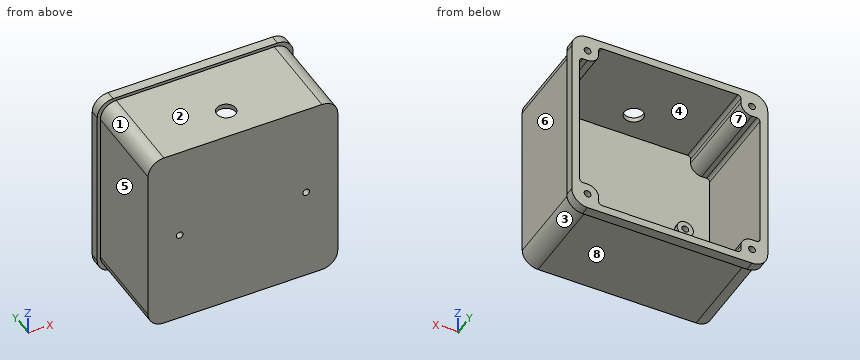
```python
from build123d import *

# Parameters (mm, degrees)
SKETCH1_W           = 120
SKETCH1_H           = 120
BOSS_EXTRUDE1_DEPTH = 63
SHELL1_T            = -3
SKETCH2_R           = 2.15
BOSS_EXTRUDE2_DEPTH = 60
SKETCH3_W           = 124
SKETCH3_H           = 124
SKETCH3_W_2         = 120
SKETCH3_H_2         = 120
BOSS_EXTRUDE3_DEPTH = 6
FILLET1_R           = 10
SKETCH4_R           = 2.15
CUT_EXTRUDE1_DEPTH  = 3
BOSS_EXTRUDE4_START = 3
SKETCH5_R           = 5.15
SKETCH5_R_2         = 2.15
BOSS_EXTRUDE4_DEPTH = 3
SKETCH6_R           = 6
CUT_EXTRUDE2_DEPTH  = 10


with BuildPart() as part:
    # Sketch1 → Boss-Extrude1 (new body)
    with BuildSketch(Plane(origin=(0, 0, 0), x_dir=(1, 0, 0), z_dir=(0, 1, 0))):
        Rectangle(SKETCH1_W, SKETCH1_H)
    extrude(amount=BOSS_EXTRUDE1_DEPTH)

    # Shell1
    shell1_openings = [part.faces().sort_by_distance(p)[0] for p in [
        (0, 63, 0),
    ]]
    offset(amount=SHELL1_T, openings=shell1_openings, kind=Kind.INTERSECTION)

    # Sketch2 → Boss-Extrude2 (add)
    # profile 1 of 4: a face of its own
    with BuildSketch(Plane(origin=(0, 3, 0), x_dir=(1, 0, 0), z_dir=(0, 1, 0))):
        with BuildLine():
            Line((52, 44.98), (55, 44.98))
            ThreePointArc((55, 44.98), (56.414213562, 44.394213562), (57, 42.98))
            Line((57, 42.98), (57, 57))
            Line((57, 57), (42.98, 57))
            ThreePointArc((42.98, 57), (44.394213562, 56.414213562), (44.98, 55))
            Line((44.98, 55), (44.98, 52))
            ThreePointArc((44.98, 52), (47.036110396, 47.036110396), (52, 44.98))
        make_face()
        with Locations(Location((52, 52, 0), (0, 0, 90))):
            Circle(SKETCH2_R, mode=Mode.SUBTRACT)
    # profile 2 of 4: a face of its own
    with BuildSketch(Plane(origin=(0, 3, 0), x_dir=(1, 0, 0), z_dir=(0, 1, 0))):
        with BuildLine():
            Line((-44.98, 52), (-44.98, 55))
            ThreePointArc((-44.98, 55), (-44.394213562, 56.414213562), (-42.98, 57))
            Line((-42.98, 57), (-57, 57))
            Line((-57, 57), (-57, 42.98))
            ThreePointArc((-57, 42.98), (-56.414213562, 44.394213562), (-55, 44.98))
            Line((-55, 44.98), (-52, 44.98))
            ThreePointArc((-52, 44.98), (-47.036110396, 47.036110396), (-44.98, 52))
        make_face()
        with Locations(Location((-52, 52, 0), (0, 0, 270))):
            Circle(SKETCH2_R, mode=Mode.SUBTRACT)
    # profile 3 of 4: a face of its own
    with BuildSketch(Plane(origin=(0, 3, 0), x_dir=(1, 0, 0), z_dir=(0, 1, 0))):
        with BuildLine():
            Line((57, -42.98), (57, -57))
            Line((57, -57), (42.98, -57))
            ThreePointArc((42.98, -57), (44.394213562, -56.414213562), (44.98, -55))
            Line((44.98, -55), (44.98, -52))
            ThreePointArc((44.98, -52), (47.036110396, -47.036110396), (52, -44.98))
            Line((52, -44.98), (55, -44.98))
            ThreePointArc((55, -44.98), (56.414213562, -44.394213562), (57, -42.98))
        make_face()
        with Locations(Location((52, -52, 0), (0, 0, 270))):
            Circle(SKETCH2_R, mode=Mode.SUBTRACT)
    # profile 4 of 4: a face of its own
    with BuildSketch(Plane(origin=(0, 3, 0), x_dir=(1, 0, 0), z_dir=(0, 1, 0))):
        with BuildLine():
            Line((-52, -44.98), (-55, -44.98))
            ThreePointArc((-55, -44.98), (-56.414213562, -44.394213562), (-57, -42.98))
            Line((-57, -42.98), (-57, -57))
            Line((-57, -57), (-42.98, -57))
            ThreePointArc((-42.98, -57), (-44.394213562, -56.414213562), (-44.98, -55))
            Line((-44.98, -55), (-44.98, -52))
            ThreePointArc((-44.98, -52), (-47.036110396, -47.036110396), (-52, -44.98))
        make_face()
        with Locations(Location((-52, -52, 0), (0, 0, 90))):
            Circle(SKETCH2_R, mode=Mode.SUBTRACT)
    extrude(amount=BOSS_EXTRUDE2_DEPTH)

    # Sketch3 → Boss-Extrude3 (add)
    with BuildSketch(Plane(origin=(0, 63, 0), x_dir=(1, 0, 0), z_dir=(0, 1, 0))):
        Rectangle(SKETCH3_W, SKETCH3_H)
        Rectangle(SKETCH3_W_2, SKETCH3_H_2, mode=Mode.SUBTRACT)
    extrude(amount=-BOSS_EXTRUDE3_DEPTH)

    # Fillet1
    fillet1_edges = [part.edges().sort_by_distance(p)[0] for p in [
        (60, 28.5, 60),
        (-60, 28.5, 60),
        (-60, 28.5, -60),
        (60, 28.5, -60),
        (62, 60, -62),
        (62, 60, 62),
        (-62, 60, 62),
        (-62, 60, -62),
    ]]
    fillet(fillet1_edges, radius=FILLET1_R)

    # Sketch4 → Cut-Extrude1 (cut)
    with BuildSketch(Plane(origin=(0, 3, 0), x_dir=(1, 0, 0), z_dir=(0, 1, 0))):
        with Locations(Location((-40, 0, 0), (0, 0, 270))):
            Circle(SKETCH4_R)
        with Locations(Location((40, 0, 0), (0, 0, 90))):
            Circle(SKETCH4_R)
    extrude(amount=-CUT_EXTRUDE1_DEPTH, mode=Mode.SUBTRACT)

    # Sketch5 → Boss-Extrude4 (add)
    # profile 1 of 2: a face of its own
    with BuildSketch(Plane(origin=(0, 3, 0), x_dir=(1, 0, 0), z_dir=(0, 1, 0)).offset(BOSS_EXTRUDE4_START)):
        with Locations(Location((-40, 0, 0), (0, 0, 270))):
            Circle(SKETCH5_R)
        with Locations(Location((-40, 0, 0), (0, 0, 270))):
            Circle(SKETCH5_R_2, mode=Mode.SUBTRACT)
    # profile 2 of 2: a face of its own
    with BuildSketch(Plane(origin=(0, 3, 0), x_dir=(1, 0, 0), z_dir=(0, 1, 0)).offset(BOSS_EXTRUDE4_START)):
        with Locations(Location((40, 0, 0), (0, 0, 90))):
            Circle(SKETCH5_R)
        with Locations(Location((40, 0, 0), (0, 0, 90))):
            Circle(SKETCH5_R_2, mode=Mode.SUBTRACT)
    extrude(amount=-BOSS_EXTRUDE4_DEPTH)

    # Sketch6 → Cut-Extrude2 (cut)
    with BuildSketch(Plane.XY.offset(60)):
        with Locations((0, 20)):
            Circle(SKETCH6_R)
    extrude(amount=-CUT_EXTRUDE2_DEPTH, mode=Mode.SUBTRACT)


solid = part.part
```
Can you work these out from the model? Positions are in its coordinate system, mm. Face numbers are marked on the shaded views. A direction names the side the tool comes from. Coordinates: 2 decimals unless noted, no trailing zeros. Order: outer loops, then holes, each group sorted by start corner. A loop starts at its lowest first (then second) coordinate and runs counter-clockwise, first axis right, second up. Notation, with made-up numbers: (30.5, 16) - (77.5, 16) arc R25 ccw to (77.5, 35) - close; hole circle Ø6 at (-26, 45.5). An arc over 180 degrees is marked (long way). Answer in a Markdown table with one row per item.
1. Suppose I cut it at A-A (z = 0). Please give me the cut outline in (x, y).
Reply:
| item | result |
|---|---|
| outline | (-62, 57) - (-60, 57) - (-60, 0) - (-42.15, 0) - (-42.15, 6) - (-45.15, 6) - (-45.15, 3) - (-57, 3) - (-57, 63) - (-62, 63) - close; (-37.85, 0) - (37.85, 0) - (37.85, 6) - (34.85, 6) - (34.85, 3) - (-34.85, 3) - (-34.85, 6) - (-37.85, 6) - close; (42.15, 0) - (60, 0) - (60, 57) - (62, 57) - (62, 63) - (57, 63) - (57, 3) - (45.15, 3) - (45.15, 6) - (42.15, 6) - close |
2. For pin 1 (1.5 mm diameter, centred on x = 53.5, y = 25.5, fed in from +Z); pin 2 (10 mm diameter, centred on y = 34, z = -7, fed in from -X); pin 3 (1 mm diameter, centred on x = -36.5, y = 26, fed in from +Z), each with a flat end and sliding along its axis, tell me the tip position at first contact or that it passes through.
Reply:
| item | result |
|---|---|
| pin 1 | stops at z = 59.61 |
| pin 2 | stops at x = -60 |
| pin 3 | stops at z = 60 |
3. Suppose I cut it at C-C (x = 10). Please give me the cut outline in (y, z).
Reply:
| item | result |
|---|---|
| outline | (0, -60) - (57, -60) - (57, -62) - (63, -62) - (63, -57) - (3, -57) - (3, 57) - (63, 57) - (63, 62) - (57, 62) - (57, 60) - (0, 60) - close |
4. If I drill on line 1 along X through (y, z) = (1.4, 0); line 2 along Z through (x, y) = (34.5, 35.5); line 3 along X through (y, z) = (34, 52), over which ranges is the centre line in solid material (lowest first)?
Reply:
| item | result |
|---|---|
| line 1 | x = -60 to -42.15, -37.85 to 37.85, 42.15 to 60 |
| line 2 | z = -60 to -57, 57 to 60 |
| line 3 | x = -59.8 to -54.15, -49.85 to -44.98, 44.98 to 49.85, 54.15 to 59.8 |
5. Suppose I cut it at B-B (x = -40). Please give me the cut outline in (y, z).
Reply:
| item | result |
|---|---|
| outline | (0, -60) - (57, -60) - (57, -62) - (63, -62) - (63, -57) - (3, -57) - (3, -5.15) - (6, -5.15) - (6, -2.15) - (0, -2.15) - close; (0, 2.15) - (6, 2.15) - (6, 5.15) - (3, 5.15) - (3, 57) - (63, 57) - (63, 62) - (57, 62) - (57, 60) - (0, 60) - close |
6. For the marked faces 1, 2, 3, 4 and 5, which set-ups out of +Z, -Z, +X, -X, +Y, -Y let a thin tool reach every point of the face, with its end or its side?
Reply:
| item | result |
|---|---|
| face 1 | +Z, -X, -Y |
| face 2 | +Z, +X, -X, -Y |
| face 3 | -Z, +X, -Y |
| face 4 | +Y |
| face 5 | +Z, -Z, -X, -Y |
7. Suppose I cut it at D-D (y = 20). Give the number of separate pieces and of enclosed holes in the cut face, and give its area (3 significant figures).
Reply:
| item | result |
|---|---|
| separate pieces | 1 |
| enclosed holes | 4 |
| area | 1,770 mm^2 |
8. If we mould it in two halves opening along Z, with no side actions, what happens to the marked faces 6, 7 and 8? For each: pulls with the +Z half, pulls with the -Z half, needs draft (parallel to the pull), parting line crosses it, or undercut.
Reply:
| item | result |
|---|---|
| face 6 | needs draft |
| face 7 | undercut |
| face 8 | pulls with the -Z half |
